```python
from build123d import *

# Parameters (mm, degrees)
SKETCH1_R           = 1.75
BOSS_EXTRUDE1_DEPTH = 3


with BuildPart() as part:
    # Sketch1 → Boss-Extrude1 (new body)
    with BuildSketch(Plane(origin=(0, 0, 0), x_dir=(1, 0, 0), z_dir=(0, 1, 0))):
        with BuildLine():
            Line((-3, 6.873863542), (-3, -6.873863542))
            ThreePointArc((-3, -6.873863542), (7.5, 0), (-3, 6.873863542))
        make_face()
        with Locations((0, 4.75)):
            Circle(SKETCH1_R, mode=Mode.SUBTRACT)
        with Locations((0, -4.75)):
            Circle(SKETCH1_R, mode=Mode.SUBTRACT)
        with Locations((4, 0)):
            Circle(SKETCH1_R, mode=Mode.SUBTRACT)
    extrude(amount=BOSS_EXTRUDE1_DEPTH)


solid = part.part
```
Could you check a few things on this model? Use its own coordinates, in mm. Give positions to 0.01 mm unless a question says otherwise; leave off trailing zeros. Loops run counter-clockwise (first coordinate to the right, second up) from the corner with the lowest first, then second, coordinate; pieces in that order, holes last. Notation, with made-up numbers: (50.5, 40.25) - (106.5, 40.25) arc R9 ccw to (106.5, 46.25) - close; hole circle Ø7 at (46, 70). An arc over 180 degrees is marked (long way). Answer in a Markdown table with one row per item. Add a question column.
Q1. If we section it at C-C (x = 4.25): List the corners of the cut face in (y, z) for me.
Q2. If we section it at D-D (y = 0.85): List the corners of the cut face in (x, z) for me.
Q3. Please list where these lines run through material, in increasing order: L1, parallel to Z at x = 0, y = 2.5; L2, parallel to X at y = 0.65, z = 4; L3, parallel to Z at x = 4, y = 0.8. Write a range as from..to.
Q4. If we section it at B-B (x = 0): List the corners of the cut face in (y, z) for me, plus the area to 3 significant figures.
Q5. We'd pull the mould along Z, two halves only. Please class faces 1 (the face through (1, 3, 0)), 2 (the face through (7.497, 1.479, 0.208)), 3 (the face through (2.25, 1.48, -0.08)): +Z half, -Z half, draft (parallel to the pull), parting line (faces both ways), or undercut.
Q6. For pin 1 (2 mm diameter, centred on x = 3.5, z = -4.5, fed in from -Y), with a flat end and sliding along its axis, tell me the tip position at first contact or that it passes through.
Q7. If we section it at A-A (z = 0): List the corners of the cut face in (x, y) for me, plus the area to 3 significant figures.
The answers:
| question | item | result |
|---|---|---|
| 1 | outline | (0, -6.18) - (3, -6.18) - (3, -1.73) - (0, -1.73) - close; (0, 1.73) - (3, 1.73) - (3, 6.18) - (0, 6.18) - close |
| 2 | outline | (-3, -6.87) arc R7.5 ccw (long way) to (-3, 6.87) - close; hole circle Ø3.5 at (0, -4.75); hole circle Ø3.5 at (0, 4.75); hole circle Ø3.5 at (4, 0) |
| 3 | L1 | z = -7.5..-6.5, -3..3, 6.5..7.5 |
| 3 | L2 | x = -3..-1.58, 1.58..6.34 |
| 3 | L3 | z = -6.34..-1.75, 1.75..6.34 |
| 4 | outline | (0, -7.5) - (3, -7.5) - (3, -6.5) - (0, -6.5) - close; (0, -3) - (3, -3) - (3, 3) - (0, 3) - close; (0, 6.5) - (3, 6.5) - (3, 7.5) - (0, 7.5) - close |
| 4 | area | 24.0 mm^2 |
| 5 | face 1 | draft |
| 5 | face 2 | parting line |
| 5 | face 3 | undercut |
| 6 | pin 1 | stops at y = 0 |
| 7 | outline | (-3, 0) - (2.25, 0) - (2.25, 3) - (-3, 3) - close; (5.75, 0) - (7.5, 0) - (7.5, 3) - (5.75, 3) - close |
| 7 | area | 21.0 mm^2 |
